Build history of the part. All positions in model axes, mm. A direction names the side the tool comes from. Round coordinates to 2 decimals unless told otherwise and drop trailing zeros. Loops run counter-clockwise (first coordinate to the right, second up) from the corner with the lowest first, then second, coordinate; pieces in that order, holes last.
from build123d import *

# Parameters (mm, degrees)
F0_W      = 12
F0_H      = 5.5
F1_DEPTH  = 1.5
F2_W      = 5.5
F2_H      = 24
F3_DEPTH  = 1.5
F4_W      = 5.5
F4_H      = 22.5
F4_H_2    = 1.5
F5_DEPTH  = 1.5
F6_W      = 5.5
F6_H      = 24
F7_DEPTH  = 1.5
F8_W      = 5.5
F8_H      = 24
F9_DEPTH  = 1.5
F10_W     = 9.5
F10_H     = 5.5
F11_DEPTH = 1.5
F12_W     = 10.5
F12_H     = 5.5
F13_DEPTH = 1.5
F14_W     = 9.5
F14_H     = 5.5
F15_DEPTH = 1.5
F16_W     = 10.5
F16_H     = 5.5
F17_DEPTH = 1.5


with BuildPart() as f1:
    # F0 (on Top) → F1 (new body)
    with BuildSketch(Plane.XY):
        with Locations((14.625001, 11.201556)):
            Rectangle(F0_W, F0_H)
        with Locations((14.625001, 5.701556)):
            Rectangle(F0_W, F0_H)
    extrude(amount=F1_DEPTH)

    # F2 (on face) → F3 (join)
    with BuildSketch(Plane.XZ.offset(-2.951556)):
        with Locations((17.875001, -10.5)):
            Rectangle(F2_W, F2_H)
    extrude(amount=F3_DEPTH)

    # F4 (on face) → F5 (join)
    with BuildSketch(Plane(origin=(8.625001, 0, 0), x_dir=(0, -1, 0), z_dir=(-1, 0, 0))):
        with Locations((-5.701556, -11.25)):
            Rectangle(F4_W, F4_H)
        with Locations((-5.701556, 0.75)):
            Rectangle(F4_W, F4_H_2)
    extrude(amount=F5_DEPTH)

    # F6 (on face) → F7 (join)
    with BuildSketch(Plane(origin=(0, 13.951556, 0), x_dir=(-1, 0, 0), z_dir=(0, 1, 0))):
        with Locations((-11.375001, -10.5)):
            Rectangle(F6_W, F6_H)
    extrude(amount=F7_DEPTH)

    # F8 (on face) → F9 (join)
    with BuildSketch(Plane.YZ.offset(20.625001)):
        with Locations((11.201556, -10.5)):
            Rectangle(F8_W, F8_H)
    extrude(amount=F9_DEPTH)

    # F10 (on face) → F11 (join)
    with BuildSketch(Plane(origin=(8.625001, 0, 0), x_dir=(0, -1, 0), z_dir=(-1, 0, 0))):
        with Locations((-9.201556, -14.25)):
            Rectangle(F10_W, F10_H)
    extrude(amount=-F11_DEPTH)

    # F12 (on face) → F13 (join)
    with BuildSketch(Plane(origin=(0, 13.951556, 0), x_dir=(-1, 0, 0), z_dir=(0, 1, 0))):
        with Locations((-15.375001, -14.25)):
            Rectangle(F12_W, F12_H)
    extrude(amount=-F13_DEPTH)

    # F14 (on face) → F15 (join)
    with BuildSketch(Plane.YZ.offset(20.625001)):
        with Locations((7.701556, -14.25)):
            Rectangle(F14_W, F14_H)
    extrude(amount=-F15_DEPTH)

    # F16 (on face) → F17 (join)
    with BuildSketch(Plane.XZ.offset(-2.951556)):
        with Locations((13.875001, -14.25)):
            Rectangle(F16_W, F16_H)
    extrude(amount=-F17_DEPTH)


solid = f1.part
(1) Slice it at A-A on x = 13.75. List the corners of the cut face in (y, z).
Responses:
outline: (2.95, -17) - (4.45, -17) - (4.45, -11.5) - (2.95, -11.5) - close; (2.95, 0) - (13.95, 0) - (13.95, -11.5) - (12.45, -11.5) - (12.45, -17) - (13.95, -17) - (13.95, -22.5) - (15.45, -22.5) - (15.45, 1.5) - (2.95, 1.5) - close
(2) Slice it at D-D on z = -20.5. List the corners of the cut face in (x, y) (3 decimals), plus the area to 3 significant figures.
Responses:
outline: (7.125, 2.952) - (8.625, 2.952) - (8.625, 8.452) - (7.125, 8.452) - close; (8.625, 13.952) - (14.125, 13.952) - (14.125, 15.452) - (8.625, 15.452) - close; (15.125, 1.452) - (20.625, 1.452) - (20.625, 2.952) - (15.125, 2.952) - close; (20.625, 8.452) - (22.125, 8.452) - (22.125, 13.952) - (20.625, 13.952) - close
area: 33.0 mm2
(3) Slice it at B-B on z = -14. List the corners of the cut face in (x, y) (3 decimals), plus the area to 3 significant figures.
Responses:
outline: (7.125, 2.952) - (15.125, 2.952) - (15.125, 1.452) - (20.625, 1.452) - (20.625, 8.452) - (22.125, 8.452) - (22.125, 13.952) - (14.125, 13.952) - (14.125, 15.452) - (8.625, 15.452) - (8.625, 8.452) - (7.125, 8.452) - close; hole (10.125, 4.452) - (19.125, 4.452) - (19.125, 12.452) - (10.125, 12.452) - close
area: 93.0 mm2
(4) Slice it at C-C on y = 10. List the corners of the cut face in (x, z) (3 decimals), plus the area to 3 significant figures.
Responses:
outline: (8.625, -17) - (10.125, -17) - (10.125, -11.5) - (8.625, -11.5) - close; (8.625, 0) - (20.625, 0) - (20.625, -11.5) - (19.125, -11.5) - (19.125, -17) - (20.625, -17) - (20.625, -22.5) - (22.125, -22.5) - (22.125, 1.5) - (8.625, 1.5) - close
area: 70.5 mm2
(5) Pin check, flat tips, straight feed: P1, Ø5.5, axis at x = 17, y = 9.5, coming from the -Z side; P2, Ø4.5, axis at y = 5.5, z = -5.5, coming from the +X side (3 decimals); P3, Ø1.6, axis at x = 18, z = -5, coming from the +Y side. Stop position of each tip, or through.
Responses:
P1: stops at z = -17
P2: stops at x = 8.625
P3: stops at y = 2.95
(6) Pull direction Z, two halves, no side cores. Call faces 1 (the face through (8.625, 6, -6)), 2 (the face through (15, 4.452, -14)), 3 (the face through (21, 11, -22.5)): +Z half, -Z half, draft (parallel to the pull), parting line (faces both ways), or undercut.
Responses:
face 1: undercut
face 2: draft
face 3: -Z half
(7) Which spindle directions (+Z, -Z, +X, -X, +Y, -Y) get a long thin tool onto all of the face, cutting with end or side? Do faces 4 (the face through (15, 13, -17)), 5 (the face through (8, 8.452, -10)), 6 (the face through (21, 8.452, -11)), 7 (the face through (8, 2.952, -10)), 8 (the face through (15, 9, 0)). Say none if no direction does.
Responses:
face 4: -Z
face 5: +Z, -Z, -X, +Y
face 6: +Z, -Z, +X, -Y
face 7: +Z, -Z, -X, -Y
face 8: none
(8) Probe line 1 (Y direction, x = 12.25, z = -14.75); line 2 (Y direction, x = 14.25, z = -13.25); line 3 (X direction, y = 4.75, z = -12.75) (3 decimals). List the from-to ranges inside material, lowest first.
Responses:
line 1: y = 2.95 to 4.45, 12.45 to 15.45
line 2: y = 2.95 to 4.45, 12.45 to 13.95
line 3: x = 7.125 to 10.125, 19.125 to 20.625
